The figure shows three views and two pictorial views of one solid part (mm, origin at its lowest corner). Answer the questions. Coordinates: 2 decimals unless noted, no trailing zeros. Write each loop counter-clockwise with the first axis right and the second up, starting at its lowest first coordinate (ties: lowest second). Pieces come first, ordered by that corner, then holes.
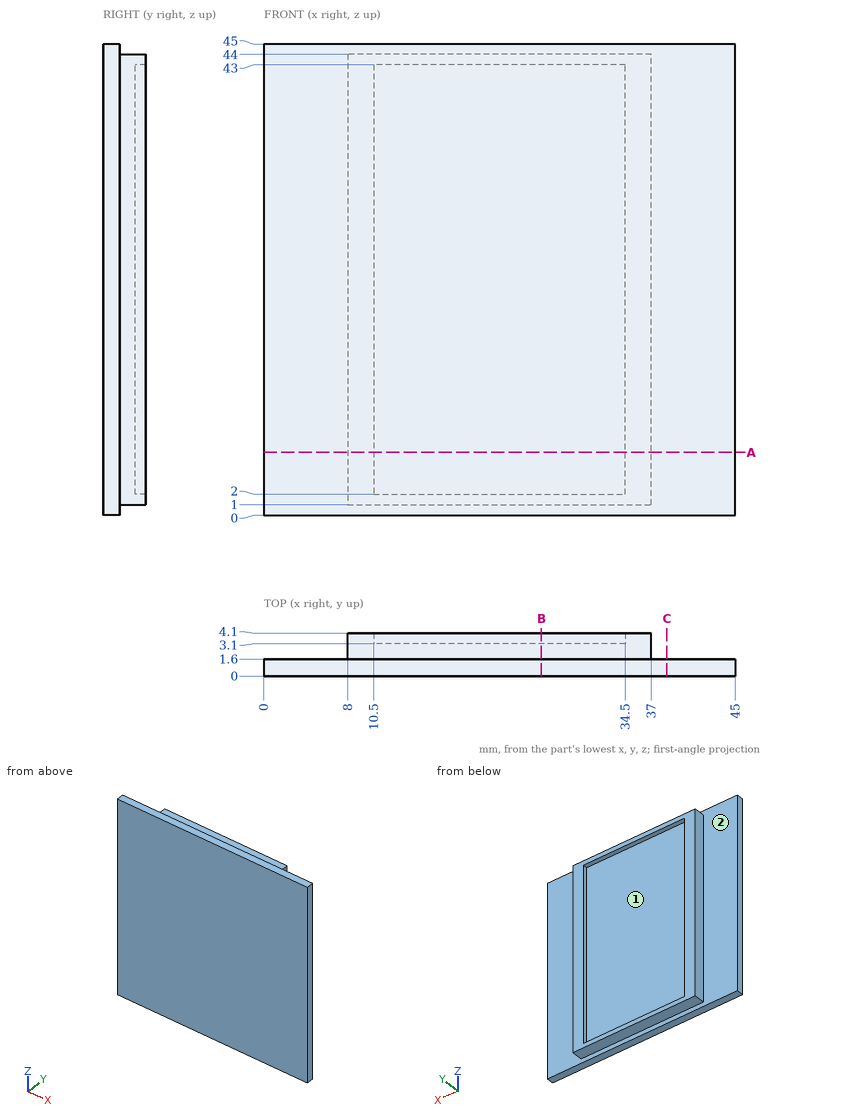
Q1. The part is cut by section C-C, the plane x = 38.5. Write down the section's boundary in (y, z).
Answers below:
outline: (0, 0) - (1.6, 0) - (1.6, 45) - (0, 45) - close
Q2. Find the intervals of material crossed by probe 1 along X at (y, z) = (3.85, 23); probe 2 along Z at (x, y) = (29.5, 3.85); probe 3 along Y at (x, z) = (23.5, 24), in increasing order.
Answers below:
probe 1: x = 8 to 10.5, 34.5 to 37
probe 2: z = 1 to 2, 43 to 44
probe 3: y = 0 to 3.1
Q3. Determine the mould class of the marked faces 1 and 2 for opening direction X: released by +X, released by -X, zero draft, split by the parting line, or undercut.
Answers below:
face 1: undercut
face 2: zero draft
Q4. Given pin 1 (2 mm diameter, centred on x = 26, y = 3, fed in from +Z); pin 2 (4 mm diameter, centred on x = 13, z = 36, fed in from +Y); pin 3 (5 mm diameter, centred on x = 22, z = 11, fed in from -Y); pin 4 (1.2 mm diameter, centred on x = 23.5, y = 2.5, fed in from -Z), each flat-ended and moving along its own axis, determine where each tip first touches the part or whether it passes through.
Answers below:
pin 1: stops at z = 44
pin 2: stops at y = 3.1
pin 3: stops at y = 0
pin 4: stops at z = 1
Q5. The part is cut by section B-B, the plane x = 26.5. Write down the section's boundary in (y, z), then the cut area to 4 significant figures.
Answers below:
outline: (0, 0) - (1.6, 0) - (1.6, 1) - (4.1, 1) - (4.1, 2) - (3.1, 2) - (3.1, 43) - (4.1, 43) - (4.1, 44) - (1.6, 44) - (1.6, 45) - (0, 45) - close
area: 138.5 mm2
Q6. The part is cut by section A-A, the plane z = 6. Write down the section's boundary in (x, y), then the cut area to 4 significant figures.
Answers below:
outline: (0, 0) - (45, 0) - (45, 1.6) - (37, 1.6) - (37, 4.1) - (34.5, 4.1) - (34.5, 3.1) - (10.5, 3.1) - (10.5, 4.1) - (8, 4.1) - (8, 1.6) - (0, 1.6) - close
area: 120.5 mm2
